```python
from build123d import *

# Parameters (mm, degrees)
F1_DEPTH = 6.35
F2_R     = 3.175
F3_R     = 6.35
F4_R     = 9.525
F5_R     = 15.875


with BuildPart() as f1:
    # F0 (on Right) → F1 (new body, symmetric)
    with BuildSketch(Plane.YZ):
        Polygon((-86.446608, 133.35), (-86.446608, 0), (-35.646608, 0), (-35.646608, 76.2), (2.453392, 76.2), (2.453392, 0), (53.253392, 0), (53.253392, 50.8), (104.053392, 50.8), (104.053392, 0), (154.853392, 0), (154.853392, 133.35), (142.153392, 133.35), (142.153392, 98.425), (-73.746608, 98.425), (-73.746608, 133.35), align=None)
    extrude(amount=F1_DEPTH, both=True)

    # F2
    f2_edges = [f1.edges().sort_by_distance(p)[0] for p in [
        (0, 53.253392, 0),
        (0, 104.053392, 0),
        (0, 2.453392, 0),
        (0, -35.646608, 0),
    ]]
    fillet(f2_edges, radius=F2_R)

    # F3
    f3_edges = [f1.edges().sort_by_distance(p)[0] for p in [
        (0, -73.746608, 98.425),
        (0, 142.153392, 98.425),
    ]]
    fillet(f3_edges, radius=F3_R)

    # F4
    f4_edges = [f1.edges().sort_by_distance(p)[0] for p in [
        (0, -73.746608, 133.35),
        (0, 142.153392, 133.35),
    ]]
    fillet(f4_edges, radius=F4_R)

    # F5
    f5_edges = [f1.edges().sort_by_distance(p)[0] for p in [
        (0, -86.446608, 0),
        (0, 154.853392, 0),
    ]]
    fillet(f5_edges, radius=F5_R)


solid = f1.part
```
Verification items for the finished model (mm, model axes). A direction names the side the tool comes from. Round coordinates to 2 decimals unless told otherwise and drop trailing zeros. Write each loop counter-clockwise with the first axis right and the second up, starting at its lowest first coordinate (ties: lowest second). Pieces come first, ordered by that corner, then holes.
1. Access from +Z, -Z, +X, -X, +Y, -Y to the whole of each face (thin tool, end or side, straight path). Record for faces 1 (the flat face through (6.35, 33, 53)), 2 (the cylindrical face through (0.089, 144.87, 130.486)), 3 (the flat face through (0, 78, 50.8)).
2. Section check B-B on x = 3. Enter the section's corners in (y, z) (3 decimals).
3. Draft check along Y on faces 4 (the cylindrical face through (0.089, -81.92, 4.774)), 5 (the cylindrical face through (-0.1, -71.9, 100.3)), 6 (the cylindrical face through (0.089, 150.326, 4.774)), 7 (the flat face through (0, 28, 0)). Enter one of: +Y half, -Y half, draft (parallel to the pull), parting line (faces both ways), or undercut.
4. Gauge pin test, flat ends, axial feed: P1, Ø4, axis at x = 0, y = 68.5, coming from the -Z side; P2, Ø4, axis at x = 1, y = -7.5, coming from the -Z side; P3, Ø5, axis at x = -1.5, y = 8.5, coming from the +Z side (3 decimals). Record the tip position at first contact, or that the pin passes through.
5. Section check A-A on z = 53.5. Enter the section's corners in (x, y), plus the area to 3 significant figures.
6. Section check C-C on z = 39. Enter the section's corners in (x, y), plus the area to 3 significant figures.
7. Section check D-D on y = -46. Enter the section's corners in (x, z) (3 decimals), plus the area to 3 significant figures.
8. Scan lines: L1, parallel to Y at x = -5.25, z = 46.5; L2, parallel to Y at x = -4.5, z = 58; L3, parallel to Y at x = 3.5, z = 119. Record each from-to range of solid material in increasing order.
Answer:
1. face 1: +Z, -Z, +X, +Y, -Y
1. face 2: +Z, +X, -X
1. face 3: -Z, +X, -X
2. outline: (-86.447, 15.875) arc R15.875 ccw to (-70.572, 0) - (-38.822, 0) arc R3.175 ccw to (-35.647, 3.175) - (-35.647, 76.2) - (2.453, 76.2) - (2.453, 3.175) arc R3.175 ccw to (5.628, 0) - (50.078, 0) arc R3.175 ccw to (53.253, 3.175) - (53.253, 50.8) - (104.053, 50.8) - (104.053, 3.175) arc R3.175 ccw to (107.228, 0) - (138.978, 0) arc R15.875 ccw to (154.853, 15.875) - (154.853, 133.35) - (151.678, 133.35) arc R9.525 ccw to (142.153, 123.825) - (142.153, 104.775) arc R6.35 cw to (135.803, 98.425) - (-67.397, 98.425) arc R6.35 cw to (-73.747, 104.775) - (-73.747, 123.825) arc R9.525 ccw to (-83.272, 133.35) - (-86.447, 133.35) - close
3. face 4: -Y half
3. face 5: undercut
3. face 6: +Y half
3. face 7: draft
4. P1: stops at z = 50.8
4. P2: stops at z = 76.2
4. P3: stops at z = 98.425
5. outline: (-6.35, -86.45) - (6.35, -86.45) - (6.35, -35.65) - (-6.35, -35.65) - close; (-6.35, 2.45) - (6.35, 2.45) - (6.35, 154.85) - (-6.35, 154.85) - close
5. area: 2,580 mm2
6. outline: (-6.35, -86.45) - (6.35, -86.45) - (6.35, -35.65) - (-6.35, -35.65) - close; (-6.35, 2.45) - (6.35, 2.45) - (6.35, 53.25) - (-6.35, 53.25) - close; (-6.35, 104.05) - (6.35, 104.05) - (6.35, 154.85) - (-6.35, 154.85) - close
6. area: 1,940 mm2
7. outline: (-6.35, 0) - (6.35, 0) - (6.35, 98.425) - (-6.35, 98.425) - close
7. area: 1,250 mm2
8. L1: y = -86.45 to -35.65, 2.45 to 53.25, 104.05 to 154.85
8. L2: y = -86.45 to -35.65, 2.45 to 154.85
8. L3: y = -86.45 to -73.75, 142.15 to 154.85
